Geometry: final body of the model. Coordinates: model frame, mm. Give positions to 0.01 mm unless a question says otherwise; leave off trailing zeros. Write each loop counter-clockwise with the first axis right and the second up, starting at its lowest first coordinate (ties: lowest second). Pieces come first, ordered by that corner, then holes. Notation, with made-up numbers: (18.25, 67.25) -> (52.25, 67.25) arc R27 cw to (52.25, 106.25) -> close; hole circle Ø6 at (82.25, -26.5). An arc over 180 degrees is marked (long way). Answer in a Markdown table with one row per item. Add a question column.
Item 1: Material intervals for probe 1 along X at (y, z) = (1.2, -30); probe 2 along X at (y, z) = (0.75, 30); probe 3 along Z at (x, y) = (-14, 4.4), sorted ascending. Write a range as from..to.
Item 2: Section query D-D on x = 53. Output: boundary loops of the cut face in (y, z), plus the area to 3 significant figures.
Item 3: Section query A-A on x = 0. Output: boundary loops of the cut face in (y, z), plus the area to 3 significant figures.
Item 4: Section query B-B on y = 3.2. State how many separate pieces and enclosed holes the cut face has, plus the area to 3 significant figures.
Item 5: Section query C-C on z = -52.5. Output: boundary loops of the cut face in (x, y).
Item 6: First-contact query: P1, Ø3.5, axis at x = -15, z = -30, coming from the -Y side; P2, Ø3, axis at y = 0.5, z = -60, coming from the +X side; P3, Ø1.8, axis at x = -15.5, y = 4, coming from the -Z side; P4, Ø2, axis at y = 1.5, z = 33.5, coming from the -X side. Flat tips, straight axial feed; report the tip coordinate or a pass-through.
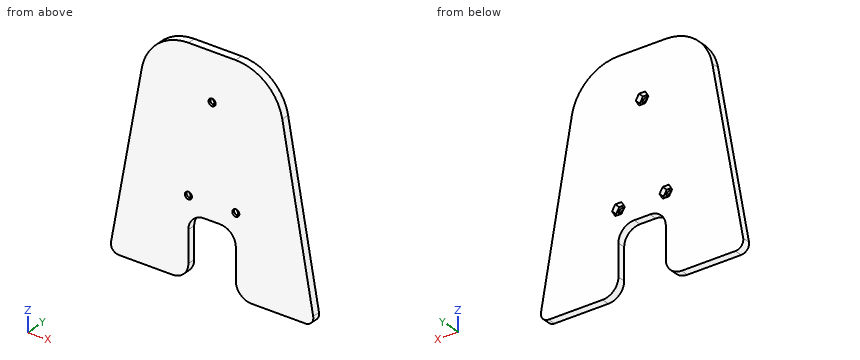
```python
from build123d import *

# Parameters (mm, degrees)
BOSS_EXTRUDE1_DEPTH = 5
SKETCH2_R           = 2.25
CUT_EXTRUDE1_DEPTH  = 5
FILLET7_R           = 30
FILLET8_R           = 30
FILLET9_R           = 10
FILLET10_R          = 10
FILLET11_R          = 10
FILLET12_R          = 10
FILLET13_R          = 5
FILLET14_R          = 5
CUT_EXTRUDE2_DEPTH  = 3.5


with BuildPart() as part:
    # Sketch1 → Boss-Extrude1 (new body)
    with BuildSketch(Plane(origin=(0, 0, 0), x_dir=(1, 0, 0), z_dir=(0, 1, 0))):
        Polygon((-15, 40), (-15, 80), (-65, 80), (-40, -60), (0, -60), (40, -60), (65, 80), (15, 80), (15, 40), align=None)
    extrude(amount=BOSS_EXTRUDE1_DEPTH)

    # Sketch2 → Cut-Extrude1 (cut)
    with BuildSketch(Plane(origin=(0, 5, 0), x_dir=(1, 0, 0), z_dir=(0, 1, 0))):
        with Locations(Location((0, -30, 0), (0, 0, 270))):
            Circle(SKETCH2_R)
        with Locations(Location((-15, 30, 0), (0, 0, 270))):
            Circle(SKETCH2_R)
        with Locations(Location((15, 30, 0), (0, 0, 270))):
            Circle(SKETCH2_R)
    extrude(amount=-CUT_EXTRUDE1_DEPTH, mode=Mode.SUBTRACT)

    # Fillet7
    fillet7_edges = [part.edges().sort_by_distance(p)[0] for p in [
        (-40, 2.5, 60),
    ]]
    fillet(fillet7_edges, radius=FILLET7_R)

    # Fillet8
    fillet8_edges = [part.edges().sort_by_distance(p)[0] for p in [
        (40, 2.5, 60),
    ]]
    fillet(fillet8_edges, radius=FILLET8_R)

    # Fillet9
    fillet9_edges = [part.edges().sort_by_distance(p)[0] for p in [
        (15, 2.5, -80),
    ]]
    fillet(fillet9_edges, radius=FILLET9_R)

    # Fillet10
    fillet10_edges = [part.edges().sort_by_distance(p)[0] for p in [
        (-15, 2.5, -80),
    ]]
    fillet(fillet10_edges, radius=FILLET10_R)

    # Fillet11
    fillet11_edges = [part.edges().sort_by_distance(p)[0] for p in [
        (15, 2.5, -40),
    ]]
    fillet(fillet11_edges, radius=FILLET11_R)

    # Fillet12
    fillet12_edges = [part.edges().sort_by_distance(p)[0] for p in [
        (-15, 2.5, -40),
    ]]
    fillet(fillet12_edges, radius=FILLET12_R)

    # Fillet13
    fillet13_edges = [part.edges().sort_by_distance(p)[0] for p in [
        (65, 2.5, -80),
    ]]
    fillet(fillet13_edges, radius=FILLET13_R)

    # Fillet14
    fillet14_edges = [part.edges().sort_by_distance(p)[0] for p in [
        (-65, 2.5, -80),
    ]]
    fillet(fillet14_edges, radius=FILLET14_R)

    # Sketch3 → Cut-Extrude2 (cut)
    with BuildSketch(Plane(origin=(0, 5, 0), x_dir=(1, 0, 0), z_dir=(0, 1, 0))):
        Polygon((-4, -30), (-2, -33.464101615), (2, -33.464101615), (4, -30), (2, -26.535898385), (-2, -26.535898385), align=None)
        Polygon((-11, 30), (-13, 33.464101615), (-17, 33.464101615), (-19, 30), (-17, 26.535898385), (-13, 26.535898385), align=None)
        Polygon((19, 30), (17, 33.464101615), (13, 33.464101615), (11, 30), (13, 26.535898385), (17, 26.535898385), align=None)
    extrude(amount=-CUT_EXTRUDE2_DEPTH, mode=Mode.SUBTRACT)


solid = part.part
```
Findings below:
| question | item | result |
|---|---|---|
| 1 | probe 1 | x = -56.07..-17.25, -12.75..12.75, 17.25..56.07 |
| 1 | probe 2 | x = -45.36..-2.25, 2.25..45.36 |
| 1 | probe 3 | z = -45.64..-33.46, -26.54..60 |
| 2 | outline | (0, -80) -> (5, -80) -> (5, -12.8) -> (0, -12.8) -> close |
| 2 | area | 336 mm^2 |
| 3 | outline | (0, -40) -> (5, -40) -> (5, 26.54) -> (1.5, 26.54) -> (1.5, 27.75) -> (0, 27.75) -> close; (0, 32.25) -> (1.5, 32.25) -> (1.5, 33.46) -> (5, 33.46) -> (5, 60) -> (0, 60) -> close |
| 3 | area | 469 mm^2 |
| 4 | separate pieces | 1 |
| 4 | enclosed holes | 3 |
| 4 | area | 13,100 mm^2 |
| 5 | outline | (-60.09, 0) -> (-15, 0) -> (-15, 5) -> (-60.09, 5) -> close; (15, 0) -> (60.09, 0) -> (60.09, 5) -> (15, 5) -> close |
| 6 | P1 | passes through |
| 6 | P2 | stops at x = 61.7 |
| 6 | P3 | stops at z = -75.1 |
| 6 | P4 | stops at x = -44.91 |
